```python
from build123d import *

# Parameters (mm, degrees)
SKETCH1_W             = 23
SKETCH1_H             = 21
EXTRUDE1_DEPTH        = 5
SKETCH2_R             = 2.15
EXTRUDE2_DEPTH        = 4.3
SKETCH3_R             = 4.5
EXTRUDE3_DEPTH        = 4.5
SKETCH4_R             = 1.25
EXTRUDE4_DEPTH        = 8
SKETCH7_W             = 12
SKETCH7_H             = 26
EXTRUDE6_DEPTH        = 5
SKETCH8_R             = 2
EXTRUDE7_DEPTH        = 4
SKETCH9_R             = 1.5
EXTRUDE8_DEPTH        = 5
FILLET2_R             = 3
M3_TAPPED_HOLE1_D     = 2.5
M3_TAPPED_HOLE1_DEPTH = 8
M3_TAPPED_HOLE1_TIP   = 0.751075774
EXTRUDE9_DEPTH        = 4
FILLET1_R             = 5
EXTRUDE10_DEPTH       = 4
FILLET3_R             = 2


with BuildPart() as part:
    # Sketch1 → Extrude1 (new body)
    with BuildSketch(Plane.XY):
        with Locations((-3.5, -4)):
            Rectangle(SKETCH1_W, SKETCH1_H)
    extrude(amount=EXTRUDE1_DEPTH)

    # Sketch2 → Extrude2 (cut)
    with BuildSketch(Plane.XY.offset(5)):
        Circle(SKETCH2_R)
    extrude(amount=-EXTRUDE2_DEPTH, mode=Mode.SUBTRACT)

    # Sketch3 → Extrude3 (cut)
    with BuildSketch(Plane(origin=(0, 0, 0), x_dir=(-1, 0, 0), z_dir=(0, 0, -1))):
        with Locations((4.9, -6.5)):
            Circle(SKETCH3_R)
    extrude(amount=-EXTRUDE3_DEPTH, mode=Mode.SUBTRACT)

    # Sketch4 → Extrude4 (cut)
    with BuildSketch(Plane.XZ.offset(14.5)):
        with Locations(Location((-12, 2.5, 0), (0, 0, 270))):
            Circle(SKETCH4_R)
        with Locations(Location((1.4, 2.5, 0), (0, 0, 270))):
            Circle(SKETCH4_R)
    extrude(amount=-EXTRUDE4_DEPTH, mode=Mode.SUBTRACT)

    # Sketch7 → Extrude6 (add)
    with BuildSketch(Plane.XY.offset(5)):
        with Locations((14, -6.5)):
            Rectangle(SKETCH7_W, SKETCH7_H)
    extrude(amount=-EXTRUDE6_DEPTH)

    # Sketch8 → Extrude7 (cut)
    with BuildSketch(Plane.XY.offset(5)):
        with Locations((17, 1.5)):
            Circle(SKETCH8_R)
    extrude(amount=-EXTRUDE7_DEPTH, mode=Mode.SUBTRACT)

    # Sketch9 → Extrude8 (cut)
    with BuildSketch(Plane.XY.offset(5)):
        with Locations((17.5, -5.5)):
            Circle(SKETCH9_R)
    extrude(amount=-EXTRUDE8_DEPTH, mode=Mode.SUBTRACT)

    # Fillet2
    fillet2_edges = [part.edges().sort_by_distance(p)[0] for p in [
        (20, 6.5, 2.5),
        (20, -19.5, 2.5),
    ]]
    fillet(fillet2_edges, radius=FILLET2_R)

    # M3 Tapped Hole1
    with Locations(Plane(origin=(-12, -14.5, 2.5), x_dir=(0, 0, -1), z_dir=(0, -1, 0))):
        with Locations((0, 0), (0, 13.4)):
            Hole(M3_TAPPED_HOLE1_D / 2, depth=M3_TAPPED_HOLE1_DEPTH)
            with Locations((0, 0, -(M3_TAPPED_HOLE1_DEPTH + M3_TAPPED_HOLE1_TIP / 2))):  # 118° drill point
                Cone(0, M3_TAPPED_HOLE1_D / 2, M3_TAPPED_HOLE1_TIP, mode=Mode.SUBTRACT)

    # Sketch11 → Extrude9 (add)
    with BuildSketch(Plane(origin=(0, 0, 0), x_dir=(-1, 0, 0), z_dir=(0, 0, -1))):
        Polygon((-8, -19.5), (-20, -19.5), (-20, 1), (-18.1, 1), (-2, -11.07), (-2, -14.5), (-8, -14.5), align=None)
    extrude(amount=EXTRUDE9_DEPTH)

    # Fillet1
    fillet1_edges = [part.edges().sort_by_distance(p)[0] for p in [
        (-15, 6.5, 2.5),
        (20, -19.5, -2),
    ]]
    fillet(fillet1_edges, radius=FILLET1_R)

    # Sketch12 → Extrude10 (cut)
    with BuildSketch(Plane(origin=(0, 0, -4), x_dir=(-1, 0, 0), z_dir=(0, 0, -1))):
        Polygon((-19.5, 1), (-19.5, -7.5), (-15.5, -7.5), (-15.5, -0.949192547), (-18.1, 1), align=None)
    extrude(amount=-EXTRUDE10_DEPTH, mode=Mode.SUBTRACT)

    # Fillet3
    fillet3_edges = [part.edges().sort_by_distance(p)[0] for p in [
        (15.5, -7.5, -2),
        (19.5, -7.5, -2),
    ]]
    fillet(fillet3_edges, radius=FILLET3_R - 0.0001)  # a hair under: the kernel refuses the full size


solid = part.part
```
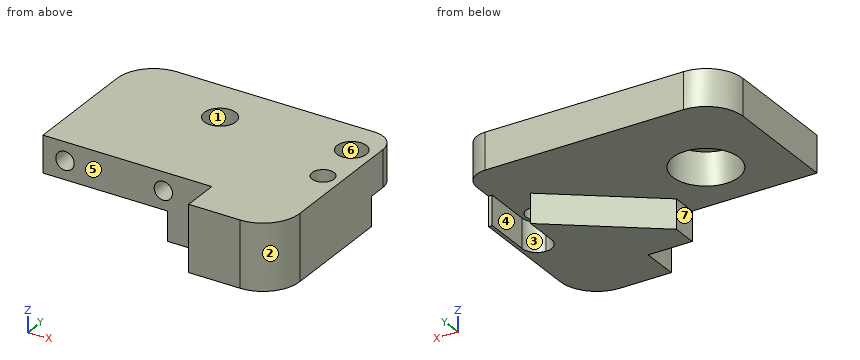
Build history of the part. All positions in model axes, mm. Face numbers are marked on the shaded views. A direction names the side the tool comes from. Give positions to 0.01 mm unless a question says otherwise; leave off trailing zeros. Loops run counter-clockwise (first coordinate to the right, second up) from the corner with the lowest first, then second, coordinate; pieces in that order, holes last. Notation, with made-up numbers: (31.25, 10) -> (80.25, 10) arc R34 cw to (80.25, 43) -> close; hole circle Ø8 at (-15.75, -14.75). An arc over 180 degrees is marked (long way). One line per question, with ' | ' between items. Start each with the question number.
1) Pin check, flat tips, straight feed: pin 1 (2.5 mm diameter, centred on x = 0, y = 0, fed in from -Z); pin 2 (2 mm diameter, centred on x = -12, z = 2.5, fed in from +Y); pin 3 (1.2 mm diameter, centred on y = -3, z = -1.5, fed in from -X); pin 4 (2.5 mm diameter, centred on x = 17.5, y = -5.5, fed in from -Z). Stop position of each tip, or through.
2) Two-plate mould, pull along Y, no slides. Class the marked faces 1, 2, 3 and 4: released by +Y, released by -Y, zero draft, split by the parting line, or undercut.
3) Probe L1, parallel to X at y = -12, z = 2.5; L2, parallel to Y at x = -4.9, z = 1.7; L3, parallel to Z at x = -12, y = -9.75. List the from-to ranges inside material, lowest first.
4) Cut at A-A (y = -13.75). Give the cut face in (x, z).
5) Cut at C-C (x = -8.5). Give the cut face in (y, z).
6) Cut at D-D (y = -3.25). Give the cut face in (x, z).
7) 3-axis set-ups, long thin cutter, end or side, ignore diameter. For the marked faces 5, 6 and 7: which of +Z, -Z, +X, -X, +Y, -Y reach the whole face in a straight line?
Return value:
1) pin 1: z = 0 | pin 2: y = 6.4 | pin 3: x = 11.96 | pin 4: through
2) face 1: undercut | face 2: released by -Y | face 3: released by +Y | face 4: zero draft
3) L1: -15 to -13.25, -10.75 to 0.15, 2.65 to 20 | L2: -14.5 to -11, -2 to 6.5 | L3: 0 to 1.25, 3.75 to 5
4) outline: (-15, 0) -> (2, 0) -> (2, -4) -> (20, -4) -> (20, 5) -> (-15, 5) -> close; hole circle Ø2.5 at (-12, 2.5); hole circle Ø2.5 at (1.4, 2.5)
5) outline: (-14.5, 0) -> (-9.2, 0) -> (-9.2, 4.5) -> (-3.8, 4.5) -> (-3.8, 0) -> (6.5, 0) -> (6.5, 5) -> (-14.5, 5) -> close
6) outline: (-15, 0) -> (-8.01, 0) -> (-8.01, 4.5) -> (-1.79, 4.5) -> (-1.79, 0) -> (12.43, 0) -> (12.43, -4) -> (15.5, -4) -> (15.5, 0) -> (19.5, 0) -> (19.5, -4) -> (20, -4) -> (20, 5) -> (-15, 5) -> close
7) face 5: +Z, -Z, -X, -Y | face 6: +Z | face 7: -Z, -X, +Y, -Y
